Source: CAD feature listing. Evaluate the final solid. Frame: model axes, mm. Face numbers are marked on the shaded views. Give positions to 0.01 mm unless a question says otherwise; leave off trailing zeros. Order: outer loops, then holes, each group sorted by start corner. A loop starts at its lowest first (then second) coordinate and runs counter-clockwise, first axis right, second up. Notation, with made-up numbers: (55.5, 0) -> (102.5, 0) arc R19 cw to (102.5, 5) -> close; hole circle Ø4 at (-22, 75.25). An arc over 180 degrees is marked (long way). Answer in a Markdown table with one row per item.
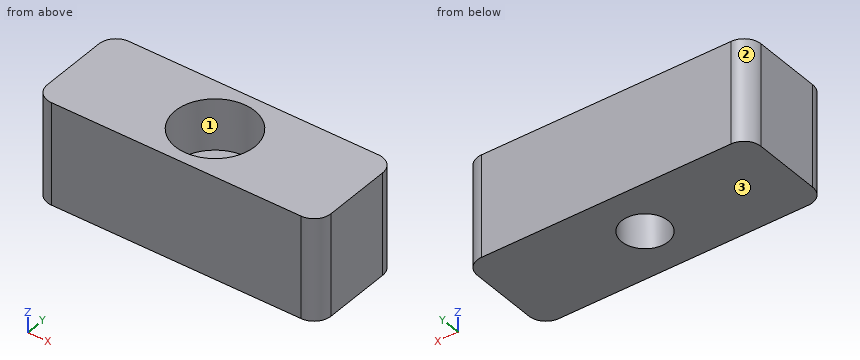
```python
from build123d import *

# Parameters (mm, degrees)
SKETCH_W     = 50
SKETCH_H     = 18
SKETCH_R     = 4.1
PAD001_DEPTH = 18
FILLET_R     = 3
SKETCH003_R  = 7
POCKET_DEPTH = 9


with BuildPart() as part:
    # Sketch → Pad001 (new body)
    with BuildSketch(Plane.XY):
        Rectangle(SKETCH_W, SKETCH_H)
        Circle(SKETCH_R, mode=Mode.SUBTRACT)
    extrude(amount=-PAD001_DEPTH)

    # Fillet
    fillet_edges = [part.edges().sort_by_distance(p)[0] for p in [
        (25, -9, -9),
        (25, 9, -9),
        (-25, 9, -9),
        (-25, -9, -9),
    ]]
    fillet(fillet_edges, radius=FILLET_R)

    # Sketch003 (on Face2 of Fillet) → Pocket (cut)
    with BuildSketch(Plane.XY):
        Circle(SKETCH003_R)
    extrude(amount=-POCKET_DEPTH, mode=Mode.SUBTRACT)


solid = part.part
```
(1) Section query B-B (y = 0). Return the cut outline in (x, z), plus the area to 3 significant figures.
A:
| item | result |
|---|---|
| outline | (-25, -18) -> (-4.1, -18) -> (-4.1, -9) -> (-7, -9) -> (-7, 0) -> (-25, 0) -> close; (4.1, -18) -> (25, -18) -> (25, 0) -> (7, 0) -> (7, -9) -> (4.1, -9) -> close |
| area | 700 mm^2 |
(2) Pull-direction query (X, two-part tool) for the marked faces 1, 2 and 3; classes: +X half, -X half, draft (parallel to the pull), parting line (faces both ways), or undercut.
A:
| item | result |
|---|---|
| face 1 | undercut |
| face 2 | -X half |
| face 3 | draft |
(3) Ray query, probe 1 along Y at (x, z) = (0, -4); probe 2 along Y at (x, z) = (0, -12.25); probe 3 along Z at (x, y) = (0, -5). Return the intervals inside material, ascending.
A:
| item | result |
|---|---|
| probe 1 | y = -9 to -7, 7 to 9 |
| probe 2 | y = -9 to -4.1, 4.1 to 9 |
| probe 3 | z = -18 to -9 |
(4) Section query A-A (x = 0). Return the cut outline in (y, z).
A:
| item | result |
|---|---|
| outline | (-9, -18) -> (-4.1, -18) -> (-4.1, -9) -> (-7, -9) -> (-7, 0) -> (-9, 0) -> close; (4.1, -18) -> (9, -18) -> (9, 0) -> (7, 0) -> (7, -9) -> (4.1, -9) -> close |
(5) Section query C-C (z = -11.75). Return the cut outline in (x, y), plus the area to 3 significant figures.
A:
| item | result |
|---|---|
| outline | (-25, -6) arc R3 ccw to (-22, -9) -> (22, -9) arc R3 ccw to (25, -6) -> (25, 6) arc R3 ccw to (22, 9) -> (-22, 9) arc R3 ccw to (-25, 6) -> close; hole circle Ø8.2 at (0, 0) |
| area | 839 mm^2 |
(6) First-contact query: pin 1 Ø7.5 at (x, y) = (0, 0) entering from -Z; pin 2 Ø6 at (x, y) = (5.5, 2.5) entering from +Z. Flat tips, straight axial feed; report the tip coordinate or a pass-through.
A:
| item | result |
|---|---|
| pin 1 | passes through |
| pin 2 | stops at z = 0 |
(7) Section query D-D (y = 4.75). Return the cut outline in (x, z), plus the area to 3 significant figures.
A:
| item | result |
|---|---|
| outline | (-25, -18) -> (25, -18) -> (25, 0) -> (5.14, 0) -> (5.14, -9) -> (-5.14, -9) -> (-5.14, 0) -> (-25, 0) -> close |
| area | 807 mm^2 |
